The listing builds one solid part. Answer for the finished solid, in the listing's coordinates (mm). Give positions to 0.01 mm unless a question says otherwise; leave off trailing zeros. Loops run counter-clockwise (first coordinate to the right, second up) from the corner with the lowest first, then second, coordinate; pieces in that order, holes last. Notation, with made-up numbers: M -29,-17 L 6,-17 A24 ccw 6,14 Z; hole C 69.5,5 d3. An arc over 180 degrees is marked long. One line per item, written item: value. Start each with the question number.
Q1. The mould has two halves that part along X. Classify faces 1 (the cylindrical face through (0, 9, 0)), 2 (the cylindrical face through (-0.33, 7.48, -0.04)), 3 (the flat face through (2, 3, 2.5)): +X half, -X half, draft (parallel to the pull), parting line (faces both ways), or undercut.
Q2. A cutting plane is placed at A-A, the plane x = 0. Determine the outline of the cut face in (y, z).
Q3. Flat-ended cylindrical pins translate along their axes: pin 1 (4 mm diameter, centred on x = 0, y = 5, fed in from +Z); pin 2 (2 mm diameter, centred on y = 7, z = -2, fed in from +X). Find the tip coordinate at first contact, or state that the pin passes through.
Q4. A cutting plane is placed at B-B, the plane z = 1.2. Determine the outline of the cut face in (x, y).
Q5. A cutting plane is placed at C-C, the plane y = 6.5. Determine the outline of the cut face in (x, z).
Q6. A cutting plane is placed at D-D, the plane x = -3. Determine the outline of the cut face in (y, z).
Q7. Consider L1, parallel to Y at x = 0, z = -0.35; L2, parallel to Y at x = 2.25, z = -0.4; L3, parallel to X at y = 7, z = -0.95. Determine where each line is inside the solid, lowest interval first.
from build123d import *

# Parameters (mm, degrees)
SKETCH1_R           = 2.5
BOSS_EXTRUDE1_DEPTH = 2.5


with BuildPart() as part:
    # Sketch1 → Boss-Extrude1 (new, symmetric)
    with BuildSketch(Plane.XY):
        with BuildLine():
            Line((-4, 0), (4, 0))
            Line((4, 0), (4, 5))
            ThreePointArc((4, 5), (0, 9), (-4, 5))
            Line((-4, 5), (-4, 0))
        make_face()
        with Locations((0, 5)):
            Circle(SKETCH1_R, mode=Mode.SUBTRACT)
    extrude(amount=BOSS_EXTRUDE1_DEPTH, both=True)


solid = part.part
Answer block:
1. face 1: parting line
1. face 2: undercut
1. face 3: draft
2. outline: M 0,-2.5 L 2.5,-2.5 L 2.5,2.5 L 0,2.5 Z; M 7.5,-2.5 L 9,-2.5 L 9,2.5 L 7.5,2.5 Z
3. pin 1: through
3. pin 2: x = 3.87
4. outline: M -4,0 L 4,0 L 4,5 A4 ccw -4,5 Z; hole C 0,5 d5
5. outline: M -3.71,-2.5 L -2,-2.5 L -2,2.5 L -3.71,2.5 Z; M 2,-2.5 L 3.71,-2.5 L 3.71,2.5 L 2,2.5 Z
6. outline: M 0,-2.5 L 7.65,-2.5 L 7.65,2.5 L 0,2.5 Z
7. L1: 0 to 2.5, 7.5 to 9
7. L2: 0 to 3.91, 6.09 to 8.31
7. L3: -3.46 to -1.5, 1.5 to 3.46
